The listing builds one solid part. Answer for the finished solid, in the listing's coordinates (mm). Coordinates: 2 decimals unless noted, no trailing zeros. Loops run counter-clockwise (first coordinate to the right, second up) from the corner with the lowest first, then second, coordinate; pieces in that order, holes last. Notation, with made-up numbers: (-32.75, 66) - (-26.75, 66) arc R15 cw to (-26.75, 78) - close; hole circle Ø10 at (51, 43.25). An arc over 180 degrees is marked (long way). Put each result on its own line as item: value.
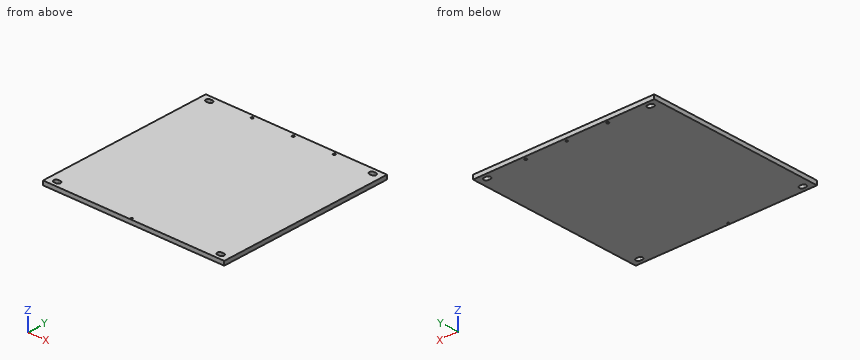
```python
from build123d import *

# Parameters (mm, degrees)
CROQUIS1_W                      = 265
CROQUIS1_H                      = 260
BRIDA_BASE1_DEPTH               = 6
RANURA_START                    = -6
RANURA_DE_MARGEN_PARA_M61_DEPTH = 6
CROQUIS5_R                      = 1.2
CORTAR_EXTRUIR1_DEPTH           = 186.72089274
TALADRO_DE_MARGEN_PARA_M31_D    = 3.4


# Read off the part's stored shape, not the designer's step: Ranura de margen para M61
# Sheet-metal steps are written as plain solids
with BuildPart() as part:
    # Croquis1 → Brida base1 (new body)
    with BuildSketch(Plane.XY):
        Rectangle(CROQUIS1_W, CROQUIS1_H)
    extrude(amount=-BRIDA_BASE1_DEPTH)

    # Ranura de margen para M61 outline → Ranura de margen para M61 (cut)
    with BuildSketch(Plane.XY.offset(RANURA_START)):
        with BuildLine():
            ThreePointArc((-118, 118), (-114.5, 121.5), (-118, 125))
            Line((-118, 125), (-121, 125))
            ThreePointArc((-121, 125), (-124.5, 121.5), (-121, 118))
            Line((-121, 118), (-118, 118))
        make_face()
        with BuildLine():
            ThreePointArc((118, 125), (114.5, 121.5), (118, 118))
            Line((118, 118), (121, 118))
            ThreePointArc((121, 118), (124.5, 121.5), (121, 125))
            Line((121, 125), (118, 125))
        make_face()
        with BuildLine():
            ThreePointArc((121, -125), (124.5, -121.5), (121, -118))
            Line((121, -118), (118, -118))
            ThreePointArc((118, -118), (114.5, -121.5), (118, -125))
            Line((118, -125), (121, -125))
        make_face()
        with BuildLine():
            ThreePointArc((-121, -118), (-124.5, -121.5), (-121, -125))
            Line((-121, -125), (-118, -125))
            ThreePointArc((-118, -125), (-114.5, -121.5), (-118, -118))
            Line((-118, -118), (-121, -118))
        make_face()
    extrude(amount=RANURA_DE_MARGEN_PARA_M61_DEPTH, mode=Mode.SUBTRACT)

    # Croquis5 → Cortar-Extruir1 (cut, through all)
    with BuildSketch(Plane.XY):
        with Locations((-5, -127.5)):
            Circle(CROQUIS5_R)
    extrude(amount=-CORTAR_EXTRUIR1_DEPTH, mode=Mode.SUBTRACT)

    # Taladro de margen para M31 (through all)
    with Locations(Plane.XY):
        with Locations((60, 125), (0, 125), (-60, 125)):
            Hole(TALADRO_DE_MARGEN_PARA_M31_D / 2)


solid = part.part
```
1) The part is cut by section A-A (y = -121.5). Give the vertices of the cut face in (x, z).
Found:
outline: (-132.5, -6) - (-124.5, -6) - (-124.5, 0) - (-132.5, 0) - close; (-114.5, -6) - (114.5, -6) - (114.5, 0) - (-114.5, 0) - close; (124.5, -6) - (132.5, -6) - (132.5, 0) - (124.5, 0) - close
2) This flat-tipped pin is pushed along its axis until it touches: pin 1 (1.9 mm diameter, centred on x = -5, y = -127.5, fed in from +Z) (1 decimal). Where does it stop, or does it pass through?
Found:
pin 1: passes through
3) Straight lines are drawn through the part: L1, parallel to Y at x = -119.5, z = -0.4; L2, parallel to Y at x = -116, z = -3.5; L3, parallel to Y at x = -60, z = -4.05. For each, find the intervals that lie inside material, in ascending order. Write a range as [from, to].
Found:
L1: y = [-130, -125], [-118, 118], [125, 130]
L2: y = [-130, -124.37], [-118.63, 118.63], [124.37, 130]
L3: y = [-130, 123.3], [126.7, 130]
